Can you work these out from the model? Positions are in its coordinate system, mm. Face numbers are marked on the shaded views. A direction names the side the tool comes from. Coordinates: 2 decimals unless noted, no trailing zeros. Loops run counter-clockwise (first coordinate to the right, second up) from the corner with the lowest first, then second, coordinate; pieces in that order, holes last. Notation, with made-up numbers: M 23.5,63 L 70.5,63 A26 ccw 70.5,97 Z; hole C 78,11.5 d11. An arc over 180 degrees is marked long. Return JSON: item names as keys, results as strings. Group by question number.
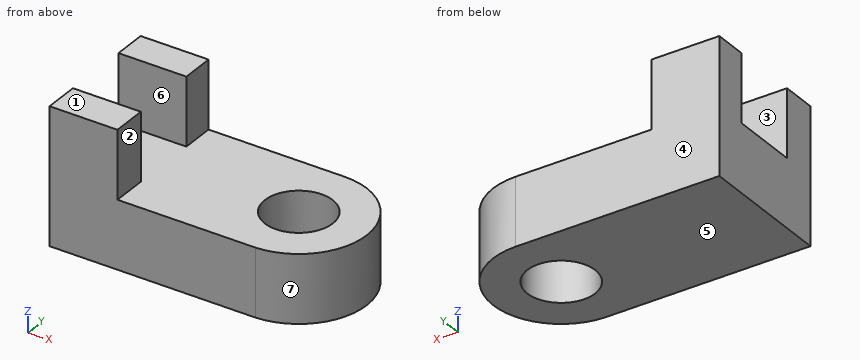
```python
from build123d import *

# Parameters (mm, degrees)
EXTRUDE1_DEPTH     = 50.8
SKETCH3_W          = 50.8
SKETCH3_H          = 101.6
EXTRUDE2_DEPTH     = 50.8
SKETCH5_W          = 50.8
SKETCH5_H          = 50.8
CUT_EXTRUDE1_DEPTH = 50.8
SKETCH6_R          = 25.4
CUT_EXTRUDE2_DEPTH = 51.8


with BuildPart() as part:
    # Sketch2 → Extrude1 (new body)
    with BuildSketch(Plane.XY):
        with BuildLine():
            Line((-68.510209021, 50.129277125), (33.089790979, 50.129277125))
            ThreePointArc((33.089790979, 50.129277125), (83.897074784, 0.175115288), (34.810357915, -51.470722875))
            Line((34.810357915, -51.470722875), (-68.510209021, -51.470722875))
            Line((-68.510209021, -51.470722875), (-68.510209021, 50.129277125))
        make_face()
    extrude(amount=EXTRUDE1_DEPTH)

    # Sketch3 → Extrude2 (add)
    with BuildSketch(Plane.ZY.offset(68.510209021)):
        with Locations((76.2, -0.670722875)):
            Rectangle(SKETCH3_W, SKETCH3_H)
        with Locations((25.4, -0.670722875)):
            Rectangle(SKETCH3_W, SKETCH3_H)
    extrude(amount=EXTRUDE2_DEPTH)

    # Sketch5 → Cut-Extrude1 (cut)
    with BuildSketch(Plane(origin=(-68.510209021, 0, 0), x_dir=(0, 0, -1), z_dir=(1, 0, 0))):
        with Locations((-76.2, -0.005051238)):
            Rectangle(SKETCH5_W, SKETCH5_H)
    extrude(amount=-CUT_EXTRUDE1_DEPTH, mode=Mode.SUBTRACT)

    # Sketch6 → Cut-Extrude2 (cut, through all)
    with BuildSketch(Plane.XY.offset(50.8)):
        with Locations((33.089790979, -0.685291529)):
            Circle(SKETCH6_R)
    extrude(amount=-CUT_EXTRUDE2_DEPTH, mode=Mode.SUBTRACT)


solid = part.part
```
1) If I drill on line 1 (X direction, y = -0.5, z = 6); line 2 (Y direction, x = -91, z = 58.5); line 3 (Z direction, x = -31, y = -2), over which ranges is the centre line in solid material (lowest first)? Write a range as from..to.
2) Suppose I cut it at D-D, the plane z = 12. List the corners of the cut face in (x, y) for me, then the cut area to 3 significant figures.
3) For pin 1 (20 mm diameter, centred on y = 43, z = 77, fed in from +X); pin 2 (1.5 mm diameter, centred on x = -40.5, y = 39, fed in from -Z); pin 3 (5 mm diameter, centred on x = -65, y = 39, fed in from +Z); pin 4 (4 mm diameter, centred on y = -32, z = 46, fed in from +X), each with a flat end and sliding along its axis, tell me the tip position at first contact or that it passes through.
4) For the marked faces 1, 2 and 3, which set-ups out of +Z, -Z, +X, -X, +Y, -Y let a thin tool reach every point of the face, with its end or its side?
5) Suppose I cut it at C-C, the plane x = -85. List the corners of the cut face in (y, z) for me.
6) Suppose I cut it at B-B, the plane y = -17. List the corners of the cut face in (x, z) for me, then the cut area to 3 significant figures.
7) Suppose I cut it at A-A, the plane z = 76.5. List the corners of the cut face in (x, y) for me, then the cut area to 3 significant figures.
8) If we mould it in two halves opening along Y, with no side actions, what happens to the marked faces 4, 5, 6 and 7? For each: +Y half, -Y half, draft (parallel to the pull), parting line (faces both ways), or undercut.
Returned:
{
 "1": {"line 1": "x = -119.31..7.69, 58.49..83.9", "line 2": "y = -51.47..-25.41, 25.39..50.13", "line 3": "z = 0..50.8"},
 "2": {"outline": "M -119.31,-51.47 L 34.81,-51.47 A50.81 ccw 33.09,50.13 L -119.31,50.13 Z; hole C 33.09,-0.69 d50.8", "area": "17,500 mm²"},
 "3": {"pin 1": "stops at x = -68.51", "pin 2": "stops at z = 0", "pin 3": "stops at z = 50.8", "pin 4": "stops at x = 74.6"},
 "4": {"face 1": "+Z, +X, -X, +Y, -Y", "face 2": "+Z, +X, +Y, -Y", "face 3": "+Z, +X, -X"},
 "5": {"outline": "M -51.47,0 L 50.13,0 L 50.13,101.6 L 25.39,101.6 L 25.39,50.8 L -25.41,50.8 L -25.41,101.6 L -51.47,101.6 Z"},
 "6": {"outline": "M -119.31,0 L 13.62,0 L 13.62,50.8 L -119.31,50.8 Z; M 52.56,0 L 81.21,0 L 81.21,50.8 L 52.56,50.8 Z", "area": "8,210 mm²"},
 "7": {"outline": "M -119.31,-51.47 L -68.51,-51.47 L -68.51,-25.41 L -119.31,-25.41 Z; M -119.31,25.39 L -68.51,25.39 L -68.51,50.13 L -119.31,50.13 Z", "area": "2,580 mm²"},
 "8": {"face 4": "+Y half", "face 5": "draft", "face 6": "undercut", "face 7": "parting line"}
}
